from build123d import *

# Parameters (mm, degrees)
SKETCH2_W           = 300
SKETCH2_H           = 300
BOSS_EXTRUDE2_DEPTH = 6


with BuildPart() as part:
    # Sketch2 → Boss-Extrude2 (new body)
    with BuildSketch(Plane(origin=(0, 0, 0), x_dir=(0, 0, -1), z_dir=(1, 0, 0))):
        Polygon((-191.5, -96.5), (-191.5, -197.5), (-101, -197.5), (-101, -191.5), (0, -191.5), (0, -197.5), (96.5, -197.5), (96.5, -191.5), (197.5, -191.5), (197.5, -101), (191.5, -101), (191.5, 0), (197.5, 0), (197.5, 96.5), (191.5, 96.5), (191.5, 197.5), (-197.5, 197.5), (-197.5, 101), (-191.5, 101), (-191.5, 0), (-197.5, 0), (-197.5, -96.5), align=None)
        Rectangle(SKETCH2_W, SKETCH2_H, mode=Mode.SUBTRACT)
    extrude(amount=BOSS_EXTRUDE2_DEPTH)


solid = part.part
Work out the finished part from the listing and answer in its coordinate system (mm). Round coordinates to 2 decimals unless told otherwise and drop trailing zeros. Order: outer loops, then holes, each group sorted by start corner. A loop starts at its lowest first (then second) coordinate and runs counter-clockwise, first axis right, second up. Notation, with made-up numbers: M 62.5,81.25 L 67.5,81.25 A20 cw 67.5,120.25 Z; hole C -7.75,75 d7. An arc over 180 degrees is marked long. One line per item, written item: value.
Q1. Find section D-D on z = -157. Write down the section's boundary in (x, y).
Derived:
outline: M 0,-191.5 L 6,-191.5 L 6,197.5 L 0,197.5 Z
Q2. Flat-ended cylindrical pins translate along their axes: pin 1 (1.8 mm diameter, centred on x = 2.5, y = -195, fed in from -Z); pin 2 (3 mm diameter, centred on x = 2, z = -193.5, fed in from -Y); pin 3 (1.8 mm diameter, centred on x = 1.5, y = 38, fed in from +Z). Find the tip coordinate at first contact, or state that the pin passes through.
Derived:
pin 1: z = -96.5
pin 2: y = -191.5
pin 3: z = 191.5
Q3. Find section A-A on x = 2.9. Write down the section's boundary in (y, z).
Derived:
outline: M -197.5,-96.5 L -191.5,-96.5 L -191.5,-197.5 L -101,-197.5 L -101,-191.5 L 0,-191.5 L 0,-197.5 L 96.5,-197.5 L 96.5,-191.5 L 197.5,-191.5 L 197.5,197.5 L 101,197.5 L 101,191.5 L 0,191.5 L 0,197.5 L -96.5,197.5 L -96.5,191.5 L -197.5,191.5 L -197.5,101 L -191.5,101 L -191.5,0 L -197.5,0 Z; hole M -150,-150 L 150,-150 L 150,150 L -150,150 Z
Q4. Straight lines are drawn through the part: line 1 (Y direction, x = 1.4, z = -85); line 2 (Z direction, x = 2.15, y = 104); line 3 (Z direction, x = 5.2, y = -121). For each, find the intervals that lie inside material, in ascending order.
Derived:
line 1: -197.5 to -150, 150 to 197.5
line 2: -191.5 to -150, 150 to 197.5
line 3: -197.5 to -150, 150 to 191.5
Q5. Find section B-B on y = -74. Write down the section's boundary in (x, z), then the cut area to 3 significant figures.
Derived:
outline: M 0,-191.5 L 6,-191.5 L 6,-150 L 0,-150 Z; M 0,150 L 6,150 L 6,197.5 L 0,197.5 Z
area: 534 mm²
